Part model, mm, in its own coordinate system. A direction names the side the tool comes from. Round coordinates to 2 decimals unless told otherwise and drop trailing zeros. Loops run counter-clockwise (first coordinate to the right, second up) from the corner with the lowest first, then second, coordinate; pieces in that order, holes last. Notation, with made-up numbers: M 32.25,75.25 L 67.25,75.25 A22 ccw 67.25,114.25 Z; hole C -22.75,81.5 d8. An arc over 180 degrees is marked long. Answer as CSV lines item,"result". Start each with the question number.
Item 1: Wall check: line 1 (Z direction, x = -23.5, y = 4); line 2 (X direction, y = 0, z = 42). Give the ranges that are in metal, low to high.
Item 2: Band-saw the part on C-C (y = -14). Give the cut face in (x, z).
Item 3: Band-saw the part on B-B (z = 5). Give the cut face in (x, y).
Item 4: Drop flat-ended pins along their axis: pin 1 Ø9.5 at (y, z) = (1, 39.5) entering from -X; pin 2 Ø9.5 at (x, y) = (-28, -2) entering from -Z; pin 3 Ø13 at (x, z) = (-25, 5.5) entering from -Y. Give the stop position or say it passes through.
Item 5: Band-saw the part on A-A (x = -1). Give the cut face in (y, z).
Item 6: Which spindle directions (+Z, -Z, +X, -X, +Y, -Y) get a long thin tool onto all of the face, cutting with end or side? Do faces 1 (the flat face through (6, -27, 7)), 2 (the flat face through (0, -27, 13.5)), 3 (the flat face through (-27, 0, 13.5)). Say none if no direction does.
```python
from build123d import *

# Parameters (mm, degrees)
SKETCH_W     = 15
SKETCH_H     = 15
PAD_DEPTH    = 15
SKETCH001_W  = 12
SKETCH001_H  = 12
PAD001_DEPTH = 40
SKETCH002_W  = 12
SKETCH002_H  = 12
PAD002_DEPTH = 40
SKETCH003_W  = 12
SKETCH003_H  = 12
PAD003_DEPTH = 40


with BuildPart() as part:
    # Sketch → Pad (new body)
    with BuildSketch(Plane.XY):
        Rectangle(SKETCH_W, SKETCH_H)
    extrude(amount=PAD_DEPTH)

    # Sketch001 → Pad001 (new body)
    with BuildSketch(Plane.XY.offset(15)):
        Rectangle(SKETCH001_W, SKETCH001_H)
    extrude(amount=PAD001_DEPTH)

    # Sketch002 → Pad002 (new body)
    with BuildSketch(Plane(origin=(-7.5, 0, 0), x_dir=(0, -1, 0), z_dir=(-1, 0, 0))):
        with Locations((0, 7.5)):
            Rectangle(SKETCH002_W, SKETCH002_H)
    extrude(amount=PAD002_DEPTH)

    # Sketch003 → Pad003 (new body)
    with BuildSketch(Plane.XZ.offset(7.5)):
        with Locations((0, 7.5)):
            Rectangle(SKETCH003_W, SKETCH003_H)
    extrude(amount=PAD003_DEPTH)


solid = part.part
```
Answer block:
1,line 1,"z = 1.5 to 13.5"
1,line 2,"x = -6 to 6"
2,outline,"M -6,1.5 L 6,1.5 L 6,13.5 L -6,13.5 Z"
3,outline,"M -47.5,-6 L -7.5,-6 L -7.5,-7.5 L -6,-7.5 L -6,-47.5 L 6,-47.5 L 6,-7.5 L 7.5,-7.5 L 7.5,7.5 L -7.5,7.5 L -7.5,6 L -47.5,6 Z"
4,pin 1,"stops at x = -6"
4,pin 2,"stops at z = 1.5"
4,pin 3,"stops at y = -6"
5,outline,"M -47.5,1.5 L -7.5,1.5 L -7.5,0 L 7.5,0 L 7.5,15 L 6,15 L 6,55 L -6,55 L -6,15 L -7.5,15 L -7.5,13.5 L -47.5,13.5 Z"
6,face 1,"+Z, -Z, +X, -Y"
6,face 2,"+Z, +X, -X, -Y"
6,face 3,"+Z, -X, +Y, -Y"
